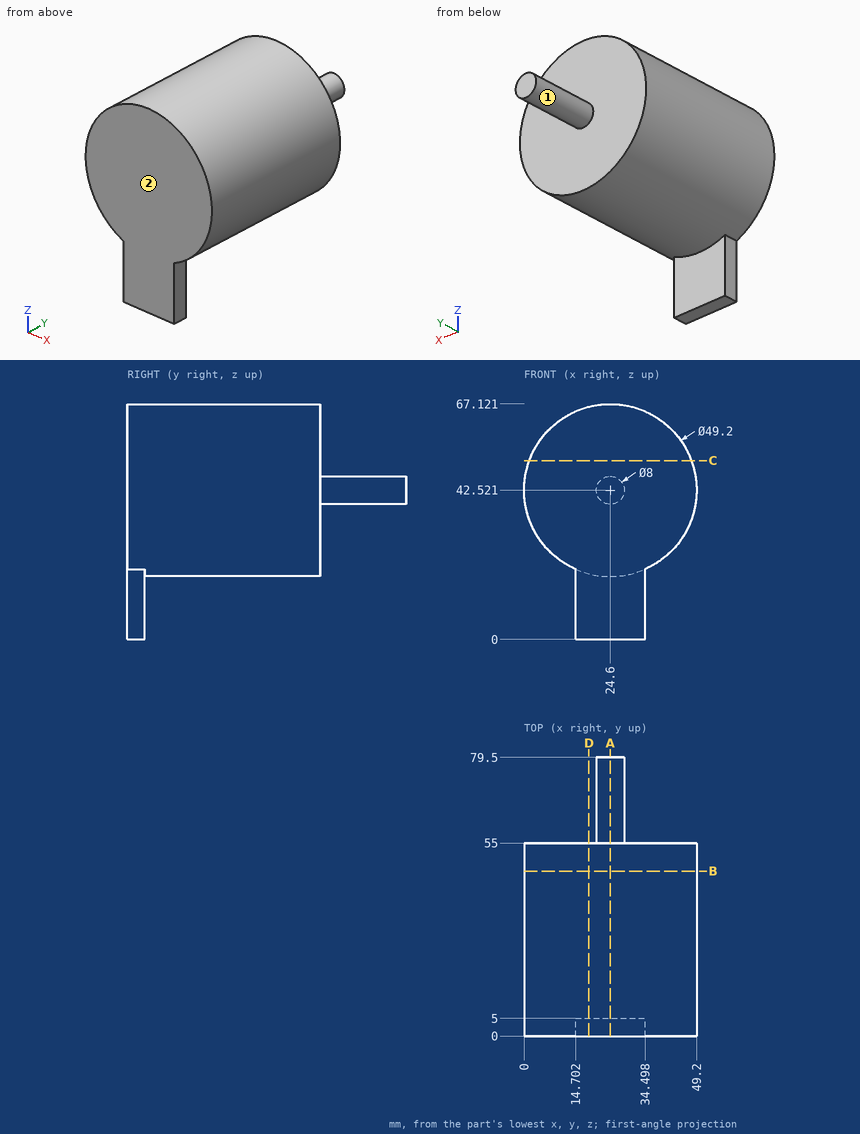
Answer from the drawing. Dimensions are ordinates in mm from the lowest x, y and z of the part. A direction names the side the tool comes from. Give positions to 0.01 mm unless a question says otherwise; leave off trailing zeros. Order: outer loops, then holes, each group sorted by start corner. A loop starts at its lowest first (then second) coordinate and runs counter-clockwise, first axis right, second up. Notation, with made-up numbers: (4, 1.25) -> (17, 1.25) arc R11 cw to (17, 19.25) -> close; hole circle Ø10 at (-39.75, 86.25). An arc over 180 degrees is marked (long way). One line per item, written item: value.
Item 1: Find section C-C, the plane z = 51. Give the vertices of the cut face in (x, y), plus the area to 3 significant figures.
Answer sheet:
outline: (1.51, 0) -> (47.69, 0) -> (47.69, 55) -> (1.51, 55) -> close
area: 2,540 mm²
Item 2: Find section A-A, the plane x = 24.6. Give the vertices of the cut face in (y, z), plus the area to 3 significant figures.
Answer sheet:
outline: (0, 0) -> (5, 0) -> (5, 17.92) -> (55, 17.92) -> (55, 38.52) -> (79.5, 38.52) -> (79.5, 46.52) -> (55, 46.52) -> (55, 67.12) -> (0, 67.12) -> close
area: 2,990 mm²
Item 3: A tool of negligible diameter and unlimited length cuts with its end or side. For the marked faces 1 and 2, from which of +Z, -Z, +X, -X, +Y, -Y can it reach the whole face along a straight path? Write none if from no direction.
Answer sheet:
face 1: +Y
face 2: +Z, -Z, +X, -X, -Y
Item 4: Find section B-B, the plane y = 47. Give the vertices of the cut face in (x, z).
Answer sheet:
outline: circle Ø49.2 at (24.6, 42.52)
Item 5: Straight lines are drawn through the part: probe 1 along Y at (x, z) = (15, 61); probe 2 along Y at (x, z) = (20.5, 8); probe 3 along Z at (x, y) = (9.5, 48). For each, find the intervals that lie inside material, in ascending order.
Answer sheet:
probe 1: 0 to 55
probe 2: 0 to 5
probe 3: 23.1 to 61.94
Item 6: Find section D-D, the plane x = 18.5. Give the vertices of the cut face in (y, z), plus the area to 4 significant figures.
Answer sheet:
outline: (0, 0) -> (5, 0) -> (5, 18.69) -> (55, 18.69) -> (55, 66.35) -> (0, 66.35) -> close
area: 2,715 mm²
Item 7: Flat-ended cylindrical pins translate along their axes: P1, Ø6, axis at y = 17, z = 34.5, coming from the -X side; P2, Ø12, axis at x = 44, y = 14.5, coming from the -Z side; P3, Ø8, axis at x = 11, z = 25.5, coming from the +Y side; P4, Ø12, axis at x = 20.5, z = 47, coming from the +Y side. Find the tip coordinate at first contact, or state that the pin passes through.
Answer sheet:
P1: x = 0.52
P2: z = 21.89
P3: y = 55
P4: y = 79.5
